Geometry: final body of the model. Coordinates: model frame, mm. Coordinates: 2 decimals unless noted, no trailing zeros. Order: outer loops, then holes, each group sorted by start corner. A loop starts at its lowest first (then second) coordinate and runs counter-clockwise, first axis right, second up. Notation, with made-up numbers: (14.5, 22) -> (54.5, 22) arc R31 ccw to (54.5, 47) -> close; hole circle Ø11 at (22.25, 57.25). An arc over 180 degrees is marked (long way). Use CSV: the item, a comma, the result in double quotes. Start each with the question number.
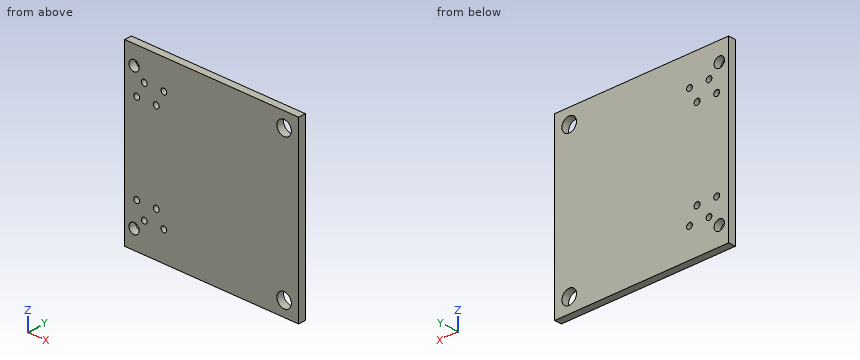
from build123d import *

# Parameters (mm, degrees)
SKETCH1_W           = 152.4
SKETCH1_H           = 152.4
SKETCH1_R           = 4.5
SKETCH1_R_2         = 2.5
SKETCH1_R_3         = 6.35
BOSS_EXTRUDE1_DEPTH = 6.35
SKETCH2_R           = 2.5527
CUT_EXTRUDE1_DEPTH  = 6.35


with BuildPart() as part:
    # Sketch1 → Boss-Extrude1 (new body)
    with BuildSketch(Plane(origin=(0, 0, 0), x_dir=(1, 0, 0), z_dir=(0, 1, 0))):
        with Locations((76.2, 76.2)):
            Rectangle(SKETCH1_W, SKETCH1_H)
        with Locations(Location((8.200009, 136.19988, 0), (0, 0, 270))):  # turned: the seam where the file's is
            Circle(SKETCH1_R, mode=Mode.SUBTRACT)
        with Locations(Location((8.200009, 16.200000112, 0), (0, 0, 270))):  # turned: the seam where the file's is
            Circle(SKETCH1_R, mode=Mode.SUBTRACT)
        with Locations(Location((17.145, 25.4, 0), (0, 0, 270))):  # turned: the seam where the file's is
            Circle(SKETCH1_R_2, mode=Mode.SUBTRACT)
        with Locations(Location((34.29, 25.4, 0), (0, 0, 270))):  # turned: the seam where the file's is
            Circle(SKETCH1_R_2, mode=Mode.SUBTRACT)
        with Locations(Location((17.145, 127, 0), (0, 0, 270))):  # turned: the seam where the file's is
            Circle(SKETCH1_R_2, mode=Mode.SUBTRACT)
        with Locations(Location((34.29, 127, 0), (0, 0, 270))):  # turned: the seam where the file's is
            Circle(SKETCH1_R_2, mode=Mode.SUBTRACT)
        with Locations(Location((139.7, 12.7, 0), (0, 0, 270))):  # turned: the seam where the file's is
            Circle(SKETCH1_R_3, mode=Mode.SUBTRACT)
        with Locations(Location((139.7, 139.7, 0), (0, 0, 270))):  # turned: the seam where the file's is
            Circle(SKETCH1_R_3, mode=Mode.SUBTRACT)
    extrude(amount=BOSS_EXTRUDE1_DEPTH)

    # Sketch2 → Cut-Extrude1 (cut)
    with BuildSketch(Plane(origin=(0, 6.35, 0), x_dir=(1, 0, 0), z_dir=(0, 1, 0))):
        with Locations(Location((10.4775, 114.3, 0), (0, 0, 270))):  # turned: the seam where the file's is
            Circle(SKETCH2_R)
        with Locations(Location((27.6225, 114.3, 0), (0, 0, 270))):  # turned: the seam where the file's is
            Circle(SKETCH2_R)
        with Locations(Location((10.4775, 38.1, 0), (0, 0, 270))):  # turned: the seam where the file's is
            Circle(SKETCH2_R)
        with Locations(Location((27.6225, 38.1, 0), (0, 0, 270))):  # turned: the seam where the file's is
            Circle(SKETCH2_R)
    extrude(amount=-CUT_EXTRUDE1_DEPTH, mode=Mode.SUBTRACT)


solid = part.part
(1) Section C-C (y = 2). State how many separate pieces and enclosed holes the cut face has, then the cut area to 3 significant figures.
(2) Line query: line 1 (Z direction, x = 134, y = 5.5); line 2 (X direction, y = 2, z = -16.2); line 3 (X direction, y = 5, z = -25.4) (3 decimals). Output: solid intervals per line, ascending. Write a range as from..to.
(3) Section B-B (z = -38.1). Return loops of the section in (x, y), then the cut area to 3 significant figures.
(4) Section A-A (x = 34.29). Return loops of the section in (y, z).
Check sheet entries:
1,separate pieces,"1"
1,enclosed holes,"12"
1,area,"22,700 mm^2"
2,line 1,"z = -152.4..-142.5, -136.9..-15.5, -9.9..0"
2,line 2,"x = 0..3.7, 12.7..134.4, 145..152.4"
2,line 3,"x = 0..14.645, 19.645..31.79, 36.79..152.4"
3,outline,"(0, 0) -> (7.92, 0) -> (7.92, 6.35) -> (0, 6.35) -> close; (13.03, 0) -> (25.07, 0) -> (25.07, 6.35) -> (13.03, 6.35) -> close; (30.18, 0) -> (152.4, 0) -> (152.4, 6.35) -> (30.18, 6.35) -> close"
3,area,"903 mm^2"
4,outline,"(0, -152.4) -> (6.35, -152.4) -> (6.35, -129.5) -> (0, -129.5) -> close; (0, -124.5) -> (6.35, -124.5) -> (6.35, -27.9) -> (0, -27.9) -> close; (0, -22.9) -> (6.35, -22.9) -> (6.35, 0) -> (0, 0) -> close"
